from build123d import *

# Parameters (mm, degrees)
PAD061_DEPTH       = 3.5
PAD059_DEPTH       = 2.5
PAD057_DEPTH       = 2
PAD058_DEPTH       = 3.5
SKETCH098_R        = 4.702209
PAD060_DEPTH       = 2.2
SKETCH099_R        = 3.711245
POCKET003044_DEPTH = 5
SKETCH101_R        = 1.7
POCKET003045_DEPTH = 5
POCKET003046_DEPTH = 3
PAD062_DEPTH       = 4


with BuildPart() as leg_link_shape:
    # Sketch100 → Pad061 (new body)
    with BuildSketch(Plane(origin=(0, 0, 31.512352), x_dir=(-1, 0, 0), z_dir=(0, 0, 1))):
        with BuildLine():
            Line((-20.438215, -2), (-13.234047, -4.102969))
            Line((-13.234047, -4.102969), (-13.028216, -6.021869))
            Line((-13.028216, -6.021869), (-13.028216, -8.298126))
            ThreePointArc((-22.034031, -8.18918), (-17.561616, -10.764285), (-13.028216, -8.298126))
            Line((-22.034031, -8.18918), (-22.034031, -2))
            Line((-20.438215, -2), (-22.034031, -2))
        make_face()
    extrude(amount=-PAD061_DEPTH)


with BuildPart() as obj1:
    # Sketch094 → Pad059 (new body)
    with BuildSketch(Plane(origin=(0, 4, 32), x_dir=(-0.981627, 0.190809, 0), z_dir=(0, 0, 1))):
        with BuildLine():
            ThreePointArc((3.75, 0.000844), (2.164719, 3.062106), (-1.25, 3.535534))
            Line((-1.25, 3.535534), (-17.000656, 2.000032))
            ThreePointArc((-17.000656, 2.000032), (-18.187877, 1.283749), (-18.711844, 0))
            ThreePointArc((-18.711844, 0), (-18.187829, -1.28373), (-17.000581, -1.999968))
            Line((-1.249867, -3.534878), (-17.000581, -1.999968))
            ThreePointArc((-1.249867, -3.534878), (2.165178, -3.061078), (3.75, 0.000844))
        make_face()
    extrude(amount=-PAD059_DEPTH)


with BuildPart() as obj2:
    # Sketch095 → Pad057 (new body, symmetric)
    with BuildSketch(Plane.XZ):
        with BuildLine():
            Line((0, 28.012352), (20.118014, 28.012352))
            ThreePointArc((27.996705, 20.985645), (25.39647, 26.000475), (20.118014, 28.012352))
            Line((27.996705, 20.985645), (30.977077, -4.999855))
            Line((33.977077, -4.999855), (30.977077, -4.999855))
            Line((31.375086, 21.001563), (33.977077, -4.999855))
            ThreePointArc((31.375086, 21.001563), (27.724484, 28.375327), (20.118014, 31.512352))
            Line((0, 31.512352), (20.118014, 31.512352))
            Line((0, 28.012352), (0, 31.512352))
        make_face()
    extrude(amount=PAD057_DEPTH, both=True)

    # Sketch096 → Pad058 (new body)
    with BuildSketch(Plane(origin=(0, 0, 31.512352), x_dir=(-1, 0, 0), z_dir=(0, 0, 1))):
        with BuildLine():
            Line((-18.002971, 2.001985), (0, 2.001985))
            ThreePointArc((0, -10), (6.000993, -3.999007), (0, 2.001985))
            Line((-19, -4), (0, -10))
            ThreePointArc((-18.002971, 2.001985), (-20.489406, -0.668781), (-19, -4))
        make_face()
    extrude(amount=-PAD058_DEPTH)

    # Cut: cut obj1
    add(obj1.part, mode=Mode.SUBTRACT)

    # Sketch098 → Pad060 (new body)
    with BuildSketch(Plane(origin=(0, 0, 28.012352), x_dir=(1, 0, 0), z_dir=(0, 0, -1))):
        with Locations((-0.089106, -3.841625)):
            Circle(SKETCH098_R)
    extrude(amount=PAD060_DEPTH)

    # Sketch099 → Pocket003044 (cut)
    with BuildSketch(Plane(origin=(0, 0, 25.812352), x_dir=(1, 0, 0), z_dir=(0, 0, -1))):
        with Locations((-0.080471, -3.899184)):
            Circle(SKETCH099_R)
    extrude(amount=-POCKET003044_DEPTH, mode=Mode.SUBTRACT)

    # Fusion007041: union leg_link_shape
    add(leg_link_shape.part)

    # Sketch101 → Pocket003045 (cut)
    with BuildSketch(Plane.XY.offset(31.512352)):
        with Locations((17.5, 6.5)):
            Circle(SKETCH101_R)
    extrude(amount=-POCKET003045_DEPTH, mode=Mode.SUBTRACT)

    # Sketch103 → Pocket003046 (cut)
    with BuildSketch(Plane.XY.offset(31.512352)):
        Polygon((18.142559, 3.16127), (20.712704, 5.387107), (20.070146, 8.725837), (16.857441, 9.83873), (14.287296, 7.612893), (14.929854, 4.274163), align=None)
    extrude(amount=-POCKET003046_DEPTH, mode=Mode.SUBTRACT)

    # Sketch102 → Pad062 (new body)
    with BuildSketch(Plane.XZ.offset(2)):
        with BuildLine():
            Line((27, 28.536497), (32.513573, -5))
            Line((32.513573, -5), (37.000002, -5))
            Line((37.000002, -5), (37.000002, -4.583553))
            ThreePointArc((33.505627, -1), (35.019116, -3.019659), (37.000002, -4.583553))
            Line((33, 5), (33.505627, -1))
            Line((35, 3.304739), (33, 5))
            Line((32.728943, 7), (35, 3.304739))
            Line((32, 13), (32.728943, 7))
            Line((34.496559, 10.608005), (32, 13))
            Line((32, 15), (34.496559, 10.608005))
            Line((31, 20), (32, 15))
            Line((33.606815, 17.606869), (31, 20))
            Line((31, 22), (33.606815, 17.606869))
            Line((27, 28.536497), (31, 22))
        make_face()
    extrude(amount=-PAD062_DEPTH)


solid = obj2.part
Can you work these out from the model? Positions are in its coordinate system, mm. A direction names the side the tool comes from. Round coordinates to 2 decimals unless told otherwise and drop trailing zeros. Order: outer loops, then holes, each group sorted by start corner. A loop starts at its lowest first (then second) coordinate and runs counter-clockwise, first axis right, second up. Notation, with made-up numbers: (-20.75, 24) - (-1.75, 24) arc R20 ccw to (-1.75, 42) - close; hole circle Ø9 at (-13, 73). An arc over 180 degrees is marked (long way). Answer in a Markdown table with one row per item.
(1) Suppose I cut it at D-D, the plane z = 25. Please give me the cut outline in (x, y).
From the geometry:
| item | result |
|---|---|
| outline | (26.34, -2) - (30.23, -2) - (30.23, 2) - (26.34, 2) - close |
(2) For P1, Ø12, axis at x = 27.5, z = 14.5, coming from the -Y side; P2, Ø6, axis at x = 3.5, y = 6.5, coming from the -Z side; P3, Ø1.5, axis at x = 14, y = 1.5, coming from the -Z side; P4, Ø18.5, axis at x = 30.5, z = 20.5, coming from the +Y side, each with a flat end and sliding along its axis, tell me the tip position at first contact or that it passes through.
From the geometry:
| item | result |
|---|---|
| P1 | stops at y = -2 |
| P2 | stops at z = 25.81 |
| P3 | stops at z = 28.01 |
| P4 | stops at y = 2 |
(3) Which directions (+Z, -Z, +X, -X, +Y, -Y) give clear straight access to the entire face, cutting with the end or side of a thin tool? Please do faces 5 (the face through (6.613, 7.912, 29.787)), 6 (the face through (4.255, 5.643, 26.928)), 7 (the face through (16.514, 3.726, 30.033)).
From the geometry:
| item | result |
|---|---|
| face 5 | +Z, -Z, +Y |
| face 6 | -Z |
| face 7 | +Z |
(4) Suppose I cut it at A-A, the plane y = 6.5. Please give me the cut outline in (x, z) (3 decimals), plus the area to 3 significant figures.
From the geometry:
| item | result |
|---|---|
| outline | (-5.455, 28.012) - (-3.968, 28.012) - (-3.968, 25.812) - (-2.728, 25.812) - (-2.728, 29.5) - (-2.795, 29.5) - (-2.795, 31.512) - (-5.455, 31.512) - close; (2.567, 25.812) - (3.79, 25.812) - (3.79, 28.012) - (11.083, 28.012) - (11.083, 31.512) - (4.36, 31.512) - (4.36, 29.5) - (2.567, 29.5) - close; (13.028, 28.012) - (15.8, 28.012) - (15.8, 28.512) - (14.501, 28.512) - (14.501, 31.512) - (13.028, 31.512) - close; (19.2, 28.012) - (22.034, 28.012) - (22.034, 31.512) - (20.499, 31.512) - (20.499, 28.512) - (19.2, 28.512) - close |
| area | 52.9 mm2 |
(5) Suppose I cut it at B-B, the plane x = -0.5. Please give me the cut outline in (y, z).
From the geometry:
| item | result |
|---|---|
| outline | (-1.98, 28.01) - (-0.84, 28.01) - (-0.84, 25.81) - (0.21, 25.81) - (0.21, 30.81) - (0.28, 30.81) - (0.28, 31.51) - (-1.98, 31.51) - close; (7.59, 25.81) - (8.53, 25.81) - (8.53, 28.01) - (9.98, 28.01) - (9.98, 31.51) - (7.72, 31.51) - (7.72, 29.5) - (7.59, 29.5) - close |
(6) If we mould it in two halves opening along Z, with no side actions, what happens to faces 1 (the face through (32, 0, -5)), 2 (the face through (32.45, -0.03, 19.56)), 3 (the face through (34.014, -0.028, 4.141)), 4 (the face through (14.604, 5.967, 30.033))? For each: released by +Z, released by -Z, zero draft, split by the parting line, or undercut.
From the geometry:
| item | result |
|---|---|
| face 1 | released by -Z |
| face 2 | released by +Z |
| face 3 | undercut |
| face 4 | zero draft |
(7) Please list where these lines run through material, in increasing order: L1, parallel to Y at x = 17.5, z = 28.15; L2, parallel to Z at x = 18.5, y = 8.75; L3, parallel to Z at x = -3, y = -0.75. Write a range as from..to.
From the geometry:
| item | result |
|---|---|
| L1 | y = -2..4.8, 8.2..10.76 |
| L2 | z = 28.01..28.51 |
| L3 | z = 28.01..31.51 |
(8) Suppose I cut it at C-C, the plane x = 23.5. Please give me the cut outline in (y, z), plus the area to 3 significant figures.
From the geometry:
| item | result |
|---|---|
| outline | (-2, 27.26) - (2, 27.26) - (2, 30.9) - (-2, 30.9) - close |
| area | 14.6 mm2 |
